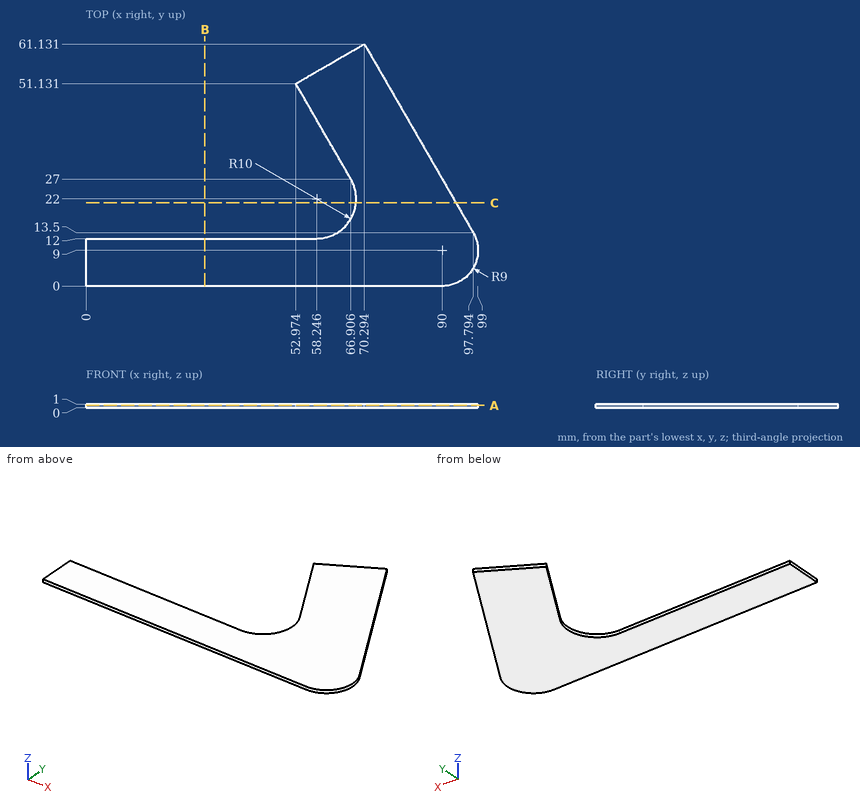
Input: dimensioned drawing with shaded views. Units: mm. Origin: part minimum x, y, z. Give positions to 0.01 mm unless a question says otherwise; leave off trailing zeros. Loops run counter-clockwise (first coordinate to the right, second up) from the corner with the lowest first, then second, coordinate; pieces in that order, holes last. Notation, with made-up numbers: (4, 62) - (29, 62) arc R14 cw to (29, 81) - close; hole circle Ø11 at (60, 21). An arc over 180 degrees is marked (long way). Answer as CSV lines item,"result". Start each with the question number.
(1) Ray query, line 1 along Y through (x, z) = (44.5, 0.9); line 2 along Y through (x, z) = (62.5, 0.3); line 3 along Y through (x, z) = (57.5, 0.6) (1 decimal). Return the intervals inside material, ascending. Write a range as [from, to].
(2) Section query C-C (y = 21). Output: boundary loops of the cut face in (x, z) (1 decimal).
(3) Section query A-A (z = 0.65). Output: boundary loops of the cut face in (x, y) (1 decimal), and give its area (3 significant figures).
(4) Section query B-B (x = 30). Output: boundary loops of the cut face in (y, z).
Worked answers:
1,line 1,"y = [0, 12]"
1,line 2,"y = [0, 12.95], [34.63, 56.63]"
1,line 3,"y = [0, 12], [43.3, 53.7]"
2,outline,"(68.2, 0) - (93.5, 0) - (93.5, 1) - (68.2, 1) - close"
3,outline,"(0, 0) - (90, 0) arc R9 ccw to (97.8, 13.5) - (70.3, 61.1) - (53, 51.1) - (66.9, 27) arc R10 cw to (58.2, 12) - (0, 12) - close"
3,area,"2,260 mm^2"
4,outline,"(0, 0) - (12, 0) - (12, 1) - (0, 1) - close"
